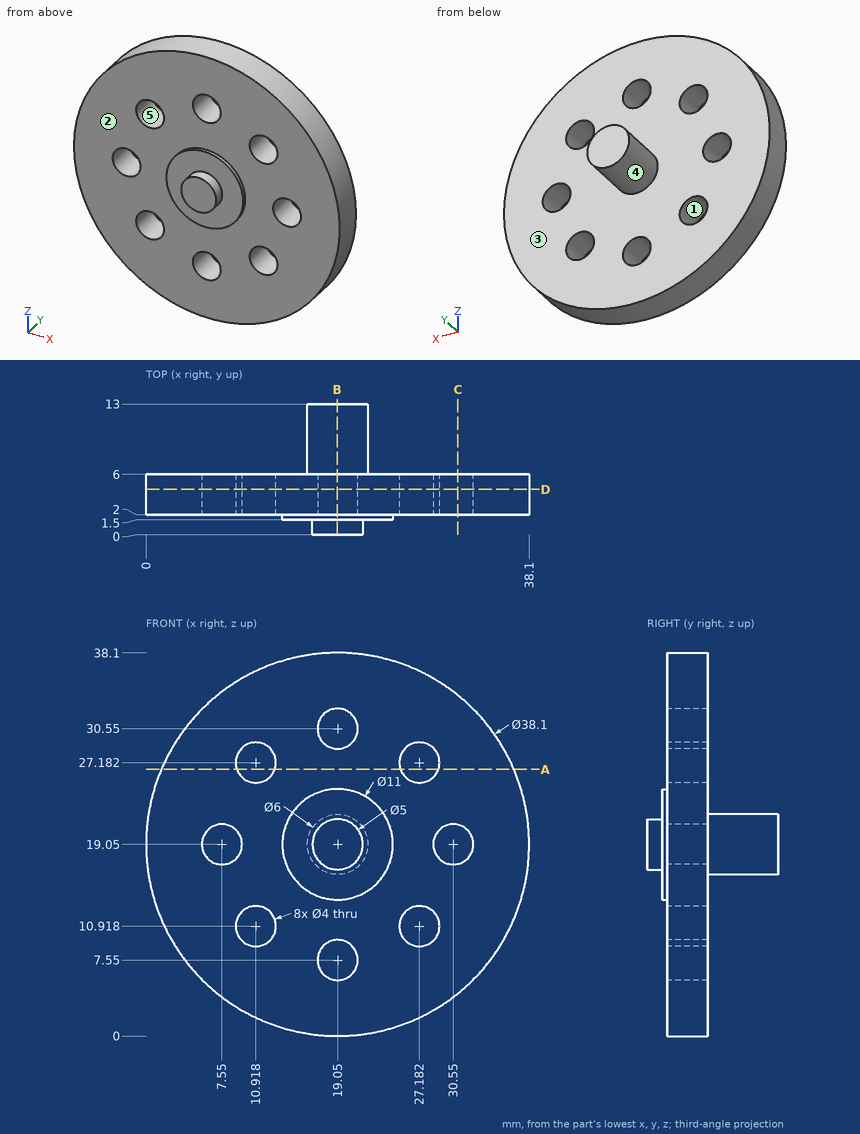
Job drawing, mm, ordinate dimensions from the low corner. One solid piece. A direction names the side the tool comes from. Give positions to 0.01 mm unless a question says otherwise; leave off trailing zeros. Loops run counter-clockwise (first coordinate to the right, second up) from the corner with the lowest first, then second, coordinate; pieces in that order, holes last. Notation, with made-up numbers: (39.5, 41.25) -> (76.5, 41.25) arc R18 cw to (76.5, 73.25) -> close; hole circle Ø7 at (17, 51). An arc over 180 degrees is marked (long way). Write each question's results on one line, items separated by ' | '. Start each with the question number.
Q1. Band-saw the part on B-B on x = 19. List the corners of the cut face in (y, z).
Q2. Which spindle directions (+Z, -Z, +X, -X, +Y, -Y) get a long thin tool onto all of the face, cutting with end or side? Do the marked faces 1 and 2. Say none if no direction does.
Q3. Band-saw the part on A-A on z = 26.5. List the corners of the cut face in (x, y).
Q4. Pin check, flat tips, straight feed: P1, Ø4, axis at x = 25.5, z = 9.5, coming from the -Y side; P2, Ø5, axis at x = 19.05, z = 7.55, coming from the +Y side; P3, Ø3.5, axis at x = 10.92, z = 10.92, coming from the -Y side; P4, Ø1.5, axis at x = 21.5, y = 8.5, coming from the -Z side. Stop position of each tip, or through.
Q5. Band-saw the part on D-D on y = 4.5. Count the separate pieces of the cut face and the enclosed holes in it, plus the area to 3 significant figures.
Q6. Band-saw the part on C-C on x = 31. List the corners of the cut face in (y, z), plus the area to 3 significant figures.
Q7. Wall check: L1, parallel to Z at x = 19, y = 3.5; L2, parallel to X at y = 4, z = 26 (1 decimal); L3, parallel to Y at x = 14, z = 4. Give the ranges that are in metal, low to high.
Q8. Pull direction Z, two halves, no side cores. Call the marked faces 3, 4 and 5: +Z half, -Z half, draft (parallel to the pull), parting line (faces both ways), or undercut.
Results are:
1) outline: (0, 16.55) -> (1.5, 16.55) -> (1.5, 13.55) -> (2, 13.55) -> (2, 9.55) -> (6, 9.55) -> (6, 16.05) -> (13, 16.05) -> (13, 22.05) -> (6, 22.05) -> (6, 28.55) -> (2, 28.55) -> (2, 24.55) -> (1.5, 24.55) -> (1.5, 21.55) -> (0, 21.55) -> close; (2, 0) -> (6, 0) -> (6, 5.55) -> (2, 5.55) -> close; (2, 32.55) -> (6, 32.55) -> (6, 38.1) -> (2, 38.1) -> close
2) face 1: +Y, -Y | face 2: -Y
3) outline: (1.52, 2) -> (9.04, 2) -> (9.04, 6) -> (1.52, 6) -> close; (12.8, 2) -> (25.3, 2) -> (25.3, 6) -> (12.8, 6) -> close; (29.06, 2) -> (36.58, 2) -> (36.58, 6) -> (29.06, 6) -> close
4) P1: stops at y = 2 | P2: stops at y = 6 | P3: passes through | P4: stops at z = 16.58
5) separate pieces: 1 | enclosed holes: 8 | area: 1,040 mm²
6) outline: (2, 4.21) -> (6, 4.21) -> (6, 17.1) -> (2, 17.1) -> close; (2, 21) -> (6, 21) -> (6, 33.89) -> (2, 33.89) -> close | area: 103 mm²
7) L1: z = 0 to 5.55, 9.55 to 28.55, 32.55 to 38.1 | L2: x = 1.3 to 9.3, 12.5 to 25.6, 28.8 to 36.8 | L3: y = 2 to 6
8) face 3: draft | face 4: parting line | face 5: undercut
